from build123d import *

# Parameters (mm, degrees)
F0_W        = 58
F0_H        = 9.5
F0_R        = 1
F0_W_2      = 44
F0_H_2      = 4.5
F1_DEPTH    = 5
F2_T1_DEPTH = 30


# Not quite as in the source:
# - a fillet or chamfer that OpenCascade refuses, or shapes differently, is made with other operations: its cross-section is extruded or revolved along the edge and cut away or added


with BuildPart() as f1:
    # F0 (on Top) → F1 (new body)
    with BuildSketch(Plane.XY):
        Rectangle(F0_W, F0_H)
        with Locations((-25.6825946271, 0)):
            Circle(F0_R, mode=Mode.SUBTRACT)
        Rectangle(F0_W_2, F0_H_2, mode=Mode.SUBTRACT)
        with Locations((25.6825946271, 0)):
            Circle(F0_R, mode=Mode.SUBTRACT)
    extrude(amount=F1_DEPTH)

    # F2: fillet of radius 5 on 4 edges, made by hand

    # F2_s2 → F2_t1 (cut)
    with BuildSketch(Plane.XY.offset(-12.5)):
        with BuildLine():
            ThreePointArc((24, -4.75), (27.5355339059, -3.2855339059), (29, 0.25))
            Line((29, 0.25), (29, -4.75))
            Line((29, -4.75), (24, -4.75))
        make_face()
        with BuildLine():
            ThreePointArc((29, -0.25), (27.5355339059, 3.2855339059), (24, 4.75))
            Line((24, 4.75), (29, 4.75))
            Line((29, 4.75), (29, -0.25))
        make_face()
        with BuildLine():
            ThreePointArc((-24, 4.75), (-27.5355339059, 3.2855339059), (-29, -0.25))
            Line((-29, -0.25), (-29, 4.75))
            Line((-29, 4.75), (-24, 4.75))
        make_face()
        with BuildLine():
            ThreePointArc((-24, -4.75), (-27.5355339059, -3.2855339059), (-29, 0.25))
            Line((-29, 0.25), (-29, -4.75))
            Line((-29, -4.75), (-24, -4.75))
        make_face()
    extrude(amount=F2_T1_DEPTH, mode=Mode.SUBTRACT)


solid = f1.part
Input: part model. Units: mm. Frame: model coordinates. A direction names the side the tool comes from. Coordinates: 2 decimals unless noted, no trailing zeros. Order: outer loops, then holes, each group sorted by start corner. A loop starts at its lowest first (then second) coordinate and runs counter-clockwise, first axis right, second up. Notation, with made-up numbers: M 21.5,33 L 50.5,33 A21 ccw 50.5,66 Z; hole C -13,-14 d5. An arc over 180 degrees is marked long. Answer in a Markdown table with one row per item.
(1) Contact query for flat-ended pins moving along their axis: pin 1 Ø3 at (y, z) = (2, 3) entering from -X; pin 2 Ø1.2 at (x, y) = (25.68, 0) entering from +Z. Output: stop coordinate, or through.
Numbers:
| item | result |
|---|---|
| pin 1 | stops at x = -28.94 |
| pin 2 | passes through |
(2) Draft query along X for faces 3 (the cylindrical face through (-24.759, -0.383, 2.465)), 4 (the cylindrical face through (27.48, 3.34, 2.46)), 5 (the cylindrical face through (-27.407, 3.409, 2.465)), 6 (the cylindrical face through (26.636, 0.3, 2.465)). Return one class per face: pulls with the +X half, pulls with the -X half, needs draft (parallel to the pull), parting line crosses it, or undercut.
Numbers:
| item | result |
|---|---|
| face 3 | undercut |
| face 4 | pulls with the +X half |
| face 5 | pulls with the -X half |
| face 6 | undercut |
(3) Material intervals for line 1 (Y direction, x = -9, z = 2.5); line 2 (X direction, y = 0.5, z = 1.6); line 3 (Y direction, x = -26.5, z = 1.6), sorted ascending. Write a range as [from, to].
Numbers:
| item | result |
|---|---|
| line 1 | y = [-4.75, -2.25], [2.25, 4.75] |
| line 2 | x = [-28.94, -26.55], [-24.82, -22], [22, 24.82], [26.55, 28.94] |
| line 3 | y = [-4.08, -0.58], [0.58, 4.08] |
(4) Section query A-A, the plane x = -10. Output: boundary loops of the cut face in (y, z).
Numbers:
| item | result |
|---|---|
| outline | M -4.75,0 L -2.25,0 L -2.25,5 L -4.75,5 Z; M 2.25,0 L 4.75,0 L 4.75,5 L 2.25,5 Z |
(5) Section query B-B, the plane z = 0.55. Output: boundary loops of the cut face in (x, y), plus the area to 3 significant figures.
Numbers:
| item | result |
|---|---|
| outline | M -28.99,0 A5 ccw -24,-4.75 L 24,-4.75 A5 ccw 28.99,0 A5 ccw 24,4.75 L -24,4.75 A5 ccw Z; hole C -25.68,0 d2; hole M -22,-2.25 L 22,-2.25 L 22,2.25 L -22,2.25 Z; hole C 25.68,0 d2 |
| area | 325 mm^2 |
(6) Access query for faces 1 (the flat face through (0, 4.75, 2)), 2 (the flat face through (-22, 0, 2)). Directions: +Z, -Z, +X, -X, +Y, -Y. A direction counts if a zero-diameter tool reaches every point of the face in a straight line with its end or side. Return the directions, or none.
Numbers:
| item | result |
|---|---|
| face 1 | +Z, -Z, +X, -X, +Y |
| face 2 | +Z, -Z |
(7) Section query D-D, the plane y = -3.75. Output: boundary loops of the cut face in (x, z), plus the area to 3 significant figures.
Numbers:
| item | result |
|---|---|
| outline | M -27,0 L 27,0 L 27,5 L -27,5 Z |
| area | 270 mm^2 |
(8) Section query C-C, the plane y = 1.75. Output: boundary loops of the cut face in (x, z).
Numbers:
| item | result |
|---|---|
| outline | M -28.58,0 L -22,0 L -22,5 L -28.58,5 Z; M 22,0 L 28.58,0 L 28.58,5 L 22,5 Z |
